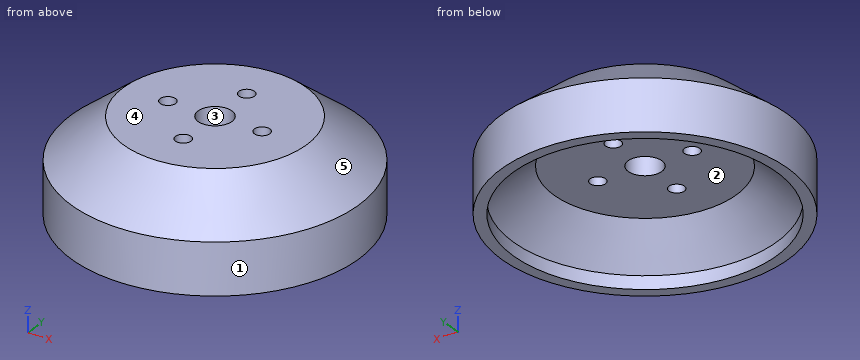
from build123d import *

# Parameters (mm, degrees)
SKETCH_1_R      = 13.5
SKETCH_1_R_2    = 1.15
SKETCH_1_R_3    = 2.5
EXTRUDE_1_DEPTH = 7


with BuildPart() as part:
    # 草图1 → 凸台-拉伸1 (new body)
    with BuildSketch(Plane.XY):
        Circle(SKETCH_1_R)
        with Locations((0, 7)):
            Circle(SKETCH_1_R_2, mode=Mode.SUBTRACT)
        with Locations((0, -7)):
            Circle(SKETCH_1_R_2, mode=Mode.SUBTRACT)
        with Locations((7, 0)):
            Circle(SKETCH_1_R_2, mode=Mode.SUBTRACT)
        with Locations((-7, 0)):
            Circle(SKETCH_1_R_2, mode=Mode.SUBTRACT)
        Circle(SKETCH_1_R_3, mode=Mode.SUBTRACT)
    extrude(amount=EXTRUDE_1_DEPTH)

    # 草图2 → 旋转1 (revolve)
    with BuildSketch(Plane(origin=(0, 0, 0), x_dir=(0, 0, -1), z_dir=(1, 0, 0)), mode=Mode.PRIVATE) as revolve_1_sk:
        Polygon((-7, 13.5), (-0.861872247, 21.199331537), (6.717890827, 21.199331537), (6.717890827, 19.5), (4.783371951, 19.5), (0, 13.5), align=None)
    revolve(revolve_1_sk.sketch.rotate(Axis((0, 0, 0), (0, 0, -1)), 90), axis=Axis((0, 0, 0), (0, 0, -1)))


solid = part.part
CAD build for the part. Positions are in the model's coordinates, mm. Face numbers are marked on the shaded views. A direction names the side the tool comes from. Give positions to 0.01 mm unless a question says otherwise; leave off trailing zeros. Order: outer loops, then holes, each group sorted by start corner. A loop starts at its lowest first (then second) coordinate and runs counter-clockwise, first axis right, second up. Notation, with made-up numbers: (-16, 44) - (36, 44) arc R20 ccw to (36, 79) - close; hole circle Ø6 at (70.5, 63). An arc over 180 degrees is marked (long way). Write each question's results on one line, items separated by ' | '.
1. Pin check, flat tips, straight feed: pin 1 (4 mm diameter, centred on x = 12, z = 4, fed in from +Y); pin 2 (1 mm diameter, centred on x = -14, z = -1.5, fed in from -Y); pin 3 (1 mm diameter, centred on x = 13.5, z = 4, fed in from +Y). Stop position of each tip, or through.
Calculated:
pin 1: stops at y = 16.04 | pin 2: stops at y = -16.35 | pin 3: stops at y = 11.9
2. Saw through at A-A on x = 0. List the corners of the cut face in (y, z), and give its area (3 significant figures).
Calculated:
outline: (-21.2, -6.72) - (-19.5, -6.72) - (-19.5, -4.78) - (-13.5, 0) - (-8.15, 0) - (-8.15, 7) - (-13.5, 7) - (-21.2, 0.86) - close; (-5.85, 0) - (-2.5, 0) - (-2.5, 7) - (-5.85, 7) - close; (2.5, 0) - (5.85, 0) - (5.85, 7) - (2.5, 7) - close; (8.15, 0) - (13.5, 0) - (19.5, -4.78) - (19.5, -6.72) - (21.2, -6.72) - (21.2, 0.86) - (13.5, 7) - (8.15, 7) - close | area: 234 mm2
3. Saw through at B-B on z = 2.5. List the corners of the cut face in (x, y), and give its area (3 significant figures).
Calculated:
outline: circle Ø38.29 at (0, 0); hole circle Ø2.3 at (-7, 0); hole circle Ø5 at (0, 0); hole circle Ø2.3 at (0, -7); hole circle Ø2.3 at (0, 7); hole circle Ø2.3 at (7, 0) | area: 1,120 mm2
4. 3-axis set-ups, long thin cutter, end or side, ignore diameter. For the marked faces 1 and 2: which of +Z, -Z, +X, -X, +Y, -Y reach the whole face in a straight line?
Calculated:
face 1: +Z, -Z | face 2: -Z
5. Pull direction X, two halves, no side cores. Call the marked faces 3, 4 and 5: released by +X, released by -X, zero draft, split by the parting line, or undercut.
Calculated:
face 3: undercut | face 4: zero draft | face 5: split by the parting line
6. Probe L1, parallel to X at y = -1, z = 2.25; L2, parallel to Z at x = -5, y = 10; L3, parallel to Y at x = 0, z = 4.5. List the from-to ranges inside material, lowest first. Write a range as from..to.
Calculated:
L1: x = -19.43..-7.57, -6.43..-2.29, 2.29..6.43, 7.57..19.43 | L2: z = 0..7 | L3: y = -16.64..-8.15, -5.85..-2.5, 2.5..5.85, 8.15..16.64
